from build123d import *

# Parameters (mm, degrees)
SKETCH1_R           = 2.35
SKETCH1_R_2         = 6.25
SKETCH1_R_3         = 2.349999999
SKETCH1_R_4         = 1.778
SKETCH1_R_5         = 1.85000011
SKETCH1_R_6         = 1.85
BOSS_EXTRUDE3_DEPTH = 6.35


with BuildPart() as part:
    # Sketch1 → Boss-Extrude3 (new body)
    with BuildSketch(Plane.XY):
        with BuildLine():
            Line((226.06, 0), (226.06, -27.287756374))
            ThreePointArc((226.06, -27.287756374), (223.084204897, -34.471961271), (215.9, -37.447756374))
            Line((215.9, -37.447756374), (-215.9, -37.447756374))
            Line((-215.9, -37.447756374), (-217.287383527, -37.447756374))
            ThreePointArc((-217.287383527, -37.447756374), (-221.777511587, -35.587884434), (-223.637383527, -31.097756374))
            Line((-223.637383527, -31.097756374), (-223.637383527, 33.765977424))
            ThreePointArc((-223.637383527, 33.765977424), (-222.309818874, 38.787300541), (-218.674059542, 42.49639313))
            Line((-218.674059542, 42.49639313), (-190.732762109, 59.128117792))
            ThreePointArc((-190.732762109, 59.128117792), (-171.969166759, 67.120649159), (-151.757691995, 69.85))
            Line((-151.757691995, 69.85), (151.757691995, 69.85))
            ThreePointArc((151.757691995, 69.85), (171.969166759, 67.120649159), (190.732762109, 59.128117792))
            Line((190.732762109, 59.128117792), (221.096676015, 41.054359515))
            ThreePointArc((221.096676015, 41.054359515), (224.732435347, 37.345266926), (226.06, 32.323943809))
            Line((226.06, 32.323943809), (226.06, 0))
        make_face()
        with Locations((-57.57418, 0)):
            Circle(SKETCH1_R, mode=Mode.SUBTRACT)
        with Locations((57.5724782, 0)):
            Circle(SKETCH1_R, mode=Mode.SUBTRACT)
        with Locations((172.72, 0)):
            Circle(SKETCH1_R, mode=Mode.SUBTRACT)
        with Locations((-115.14709, 27.952818)):
            Circle(SKETCH1_R_2, mode=Mode.SUBTRACT)
        with Locations((-0.0008509, 27.951954786)):
            Circle(SKETCH1_R_2, mode=Mode.SUBTRACT)
        with Locations((115.1462391, 27.951065379)):
            Circle(SKETCH1_R_3, mode=Mode.SUBTRACT)
        with Locations((-108.14709, 43.452818)):
            Circle(SKETCH1_R_4, mode=Mode.SUBTRACT)
        with Locations((-94.723696241, 35.702818)):
            Circle(SKETCH1_R_4, mode=Mode.SUBTRACT)
        with Locations((-94.723696241, 20.202818)):
            Circle(SKETCH1_R_4, mode=Mode.SUBTRACT)
        with Locations((-108.14709, 12.452818)):
            Circle(SKETCH1_R_4, mode=Mode.SUBTRACT)
        with Locations((-121.570483759, 20.202818)):
            Circle(SKETCH1_R_4, mode=Mode.SUBTRACT)
        with Locations((-121.570483759, 35.702818)):
            Circle(SKETCH1_R_4, mode=Mode.SUBTRACT)
        with Locations((-7.0008509, 43.451954786)):
            Circle(SKETCH1_R_4, mode=Mode.SUBTRACT)
        with Locations((6.422542859, 35.701954786)):
            Circle(SKETCH1_R_4, mode=Mode.SUBTRACT)
        with Locations((6.422542859, 20.201954786)):
            Circle(SKETCH1_R_4, mode=Mode.SUBTRACT)
        with Locations((-7.0008509, 12.451954786)):
            Circle(SKETCH1_R_4, mode=Mode.SUBTRACT)
        with Locations((-20.424244659, 20.201954786)):
            Circle(SKETCH1_R_4, mode=Mode.SUBTRACT)
        with Locations((-20.424244659, 35.701954786)):
            Circle(SKETCH1_R_4, mode=Mode.SUBTRACT)
        with Locations((-71.417984205, 64.270384182)):
            Circle(SKETCH1_R_5, mode=Mode.SUBTRACT)
        with Locations((-32.17418, 60.325)):
            Circle(SKETCH1_R_6, mode=Mode.SUBTRACT)
        with Locations((-152.82418, 60.325)):
            Circle(SKETCH1_R_6, mode=Mode.SUBTRACT)
        with Locations((152.82418, 60.325)):
            Circle(SKETCH1_R_6, mode=Mode.SUBTRACT)
        with Locations((32.17418, 60.325)):
            Circle(SKETCH1_R_6, mode=Mode.SUBTRACT)
        with Locations((-44.232364205, 64.270384182)):
            Circle(SKETCH1_R_5, mode=Mode.SUBTRACT)
        with Locations((115.1453882, -9.897181959)):
            Circle(SKETCH1_R_6, mode=Mode.SUBTRACT)
        with Locations((-115.14709, -9.897181959)):
            Circle(SKETCH1_R_6, mode=Mode.SUBTRACT)
        with Locations((-0.00127, -9.897181959)):
            Circle(SKETCH1_R_6, mode=Mode.SUBTRACT)
        with Locations((220.058830169, 33.81345012)):
            Circle(SKETCH1_R_6, mode=Mode.SUBTRACT)
        with Locations((-220.058830169, 33.81345012)):
            Circle(SKETCH1_R_6, mode=Mode.SUBTRACT)
        with Locations((220.058830169, -31.752755237)):
            Circle(SKETCH1_R_5, mode=Mode.SUBTRACT)
        with Locations((-220.000076831, -31.65099147)):
            Circle(SKETCH1_R_5, mode=Mode.SUBTRACT)
        with Locations((-71.417984205, 37.329615818)):
            Circle(SKETCH1_R_5, mode=Mode.SUBTRACT)
        with Locations((-44.232364205, 37.329615818)):
            Circle(SKETCH1_R_5, mode=Mode.SUBTRACT)
        with Locations((42.882015795, 64.270384182)):
            Circle(SKETCH1_R_5, mode=Mode.SUBTRACT)
        with Locations((70.067635795, 64.270384182)):
            Circle(SKETCH1_R_5, mode=Mode.SUBTRACT)
        with Locations((42.882015795, 37.329615818)):
            Circle(SKETCH1_R_5, mode=Mode.SUBTRACT)
        with Locations((70.067635795, 37.329615818)):
            Circle(SKETCH1_R_5, mode=Mode.SUBTRACT)
        with Locations((-128.567984205, -4.927372192)):
            Circle(SKETCH1_R_5, mode=Mode.SUBTRACT)
        with Locations((-101.382364205, -4.927372192)):
            Circle(SKETCH1_R_5, mode=Mode.SUBTRACT)
        with Locations((-101.382364205, -31.868140555)):
            Circle(SKETCH1_R_5, mode=Mode.SUBTRACT)
        with Locations((-128.567984205, -31.868140555)):
            Circle(SKETCH1_R_5, mode=Mode.SUBTRACT)
        with Locations((-14.267984205, -4.927372192)):
            Circle(SKETCH1_R_5, mode=Mode.SUBTRACT)
        with Locations((12.917635795, -4.927372192)):
            Circle(SKETCH1_R_5, mode=Mode.SUBTRACT)
        with Locations((12.917635795, -31.868140555)):
            Circle(SKETCH1_R_5, mode=Mode.SUBTRACT)
        with Locations((-14.267984205, -31.868140555)):
            Circle(SKETCH1_R_5, mode=Mode.SUBTRACT)
        with Locations((100.032015795, -4.927372192)):
            Circle(SKETCH1_R_5, mode=Mode.SUBTRACT)
        with Locations((127.217635795, -4.927372192)):
            Circle(SKETCH1_R_5, mode=Mode.SUBTRACT)
        with Locations((127.217635795, -31.868140555)):
            Circle(SKETCH1_R_5, mode=Mode.SUBTRACT)
        with Locations((100.032015795, -31.868140555)):
            Circle(SKETCH1_R_5, mode=Mode.SUBTRACT)
        with Locations((195.527631613, 45.220384182)):
            Circle(SKETCH1_R_4, mode=Mode.SUBTRACT)
        with Locations((222.468399976, 26.170384182)):
            Circle(SKETCH1_R_4, mode=Mode.SUBTRACT)
        with Locations((222.468399976, -19.820384182)):
            Circle(SKETCH1_R_4, mode=Mode.SUBTRACT)
        with Locations((195.527631613, -30.979615818)):
            Circle(SKETCH1_R_4, mode=Mode.SUBTRACT)
        with Locations((222.468399976, -0.770384182)):
            Circle(SKETCH1_R_4, mode=Mode.SUBTRACT)
        with Locations((-177.581600024, 56.379615818)):
            Circle(SKETCH1_R_4, mode=Mode.SUBTRACT)
        with Locations((-204.522368387, 45.220384182)):
            Circle(SKETCH1_R_4, mode=Mode.SUBTRACT)
        with Locations((-197.966781419, -32.314797213)):
            Circle(SKETCH1_R_4, mode=Mode.SUBTRACT)
        with Locations((-204.522368387, -19.820384182)):
            Circle(SKETCH1_R_4, mode=Mode.SUBTRACT)
        with Locations((-204.522368387, 26.170384182)):
            Circle(SKETCH1_R_4, mode=Mode.SUBTRACT)
    extrude(amount=BOSS_EXTRUDE3_DEPTH)


solid = part.part
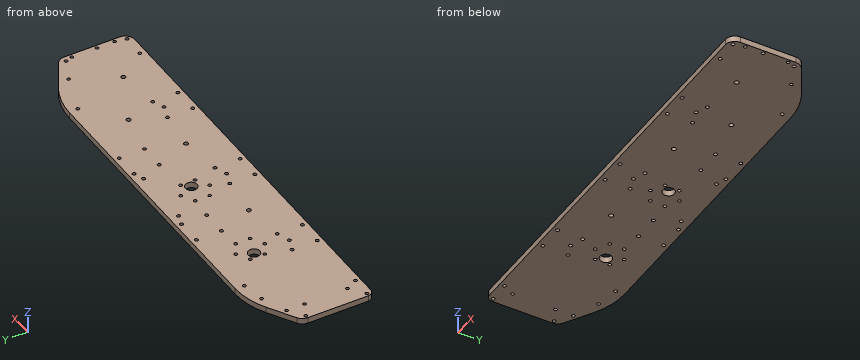
Could you check a few things on this model? Use its own coordinates, in mm. Coordinates: 2 decimals unless noted, no trailing zeros. Order: outer loops, then holes, each group sorted by start corner. A loop starts at its lowest first (then second) coordinate and runs counter-clockwise, first axis right, second up. Notation, with made-up numbers: (63.5, -6.5) -> (122.5, -6.5) arc R35 ccw to (122.5, 27.5) -> close; hole circle Ø6 at (-35.75, -12). An arc over 180 degrees is marked (long way). One line per item, written item: value. Start each with the question number.
1) If I drill on L1, parallel to Y at x = -108.5, z = 2.5; L2, parallel to X at y = -19.5, z = 2; L3, parallel to X at y = 19, z = 2, over which ranges is the centre line in solid material (lowest first)? Write a range as [from, to].
2) I'm going to push flat-ended pins straight in: pin 1 (3 mm diameter, centred on x = 115.15, y = 27.95, fed in from +Z); pin 2 (1 mm diameter, centred on x = -159, z = 3.5, fed in from +Y). Where does each tip first touch, or does it pass through?
3) Imagine slicing it at B-B on z = 3.25. Count the separate pieces of the cut face and the enclosed holes in it, plus the area to 3 significant figures.
4) Imagine slicing it at C-C on x = 184. List the corners of the cut face in (y, z) for me, plus the area to 3 significant figures.
5) Imagine slicing it at A-A on x = -170.5. List the corners of the cut face in (y, z) for me.
Answer list:
1. L1: y = [-37.45, 10.71], [14.2, 41.71], [45.2, 69.85]
1. L2: x = [-223.64, -206.27], [-202.77, 220.72], [224.22, 226.06]
1. L3: x = [-223.64, -122.88], [-120.26, -96.03], [-93.41, -21.73], [-19.11, 5.11], [7.73, 226.06]
2. pin 1: passes through
2. pin 2: stops at y = 69.55
3. separate pieces: 1
3. enclosed holes: 59
3. area: 45,600 mm2
4. outline: (-37.45, 0) -> (62.69, 0) -> (62.69, 6.35) -> (-37.45, 6.35) -> close
4. area: 636 mm2
5. outline: (-37.45, 0) -> (67.51, 0) -> (67.51, 6.35) -> (-37.45, 6.35) -> close
